For this review, take the finished solid that the model builds, in its own axes (mm). A direction names the side the tool comes from. Round coordinates to 2 decimals unless told otherwise and drop trailing zeros. Answer in a Markdown table with one row per item.
```python
from build123d import *

# Parameters (mm, degrees)
BOSS_EXTRUDE1_DEPTH     = 76.2
CUT_EXTRUDE1_DEPTH      = 79.288057838
CUT_EXTRUDE1_DEPTH_BACK = 79.288057838
SKETCH5_R               = 0.55245
SKETCH6_R               = 2.6035
CUT_EXTRUDE3_DEPTH      = 42.418


with BuildPart() as part:
    # Sketch4 → Boss-Extrude1 (new, symmetric)
    with BuildSketch(Plane.XY):
        with BuildLine():
            Line((4.190365, -12.7), (10.11729625, -12.7))
            ThreePointArc((10.11729625, -12.7), (11.943543585, -11.943543585), (12.7, -10.11729625))
            Line((12.7, -10.11729625), (12.7, -4.190365))
            ThreePointArc((12.7, -4.190365), (12.42492494, -3.52627506), (11.760835, -3.2512))
            Line((11.760835, -3.2512), (11.429365, -3.2512))
            ThreePointArc((11.429365, -3.2512), (10.76527506, -3.52627506), (10.4902, -4.190365))
            Line((10.4902, -4.190365), (10.4902, -6.348478019))
            ThreePointArc((10.4902, -6.348478019), (9.830707141, -7.335478831), (8.666460301, -7.103895736))
            Line((8.666460301, -7.103895736), (5.299899128, -3.737334563))
            ThreePointArc((5.299899128, -3.737334563), (4.817571085, -3.015479634), (4.6482, -2.16399369))
            Line((4.6482, -2.16399369), (4.6482, 0))
            Line((4.6482, 0), (2.6035, 0))
            ThreePointArc((2.6035, 0), (1.840952505, -1.840952505), (0, -2.6035))
            Line((0, -2.6035), (0, -4.6482))
            Line((0, -4.6482), (2.16399369, -4.6482))
            ThreePointArc((2.16399369, -4.6482), (3.015479634, -4.817571085), (3.737334563, -5.299899128))
            Line((3.737334563, -5.299899128), (7.103895736, -8.666460301))
            ThreePointArc((7.103895736, -8.666460301), (7.335478831, -9.830707141), (6.348478019, -10.4902))
            Line((6.348478019, -10.4902), (4.190365, -10.4902))
            ThreePointArc((4.190365, -10.4902), (3.52627506, -10.76527506), (3.2512, -11.429365))
            Line((3.2512, -11.429365), (3.2512, -11.760835))
            ThreePointArc((3.2512, -11.760835), (3.52627506, -12.42492494), (4.190365, -12.7))
        make_face()
    extrude(amount=BOSS_EXTRUDE1_DEPTH, both=True)

    # Sketch5 → Cut-Extrude1 (cut, two sides: drawn at the far end of the back side and taken through both)
    with BuildSketch(Plane.XY.offset(-CUT_EXTRUDE1_DEPTH_BACK)):
        with Locations((10.356153152, -12.7)):
            Circle(SKETCH5_R)
        with Locations((5.796028019, -12.7)):
            Circle(SKETCH5_R)
        with Locations((12.7, -10.356153152)):
            Circle(SKETCH5_R)
        with Locations((12.7, -5.796028019)):
            Circle(SKETCH5_R)
    extrude(amount=CUT_EXTRUDE1_DEPTH + CUT_EXTRUDE1_DEPTH_BACK, mode=Mode.SUBTRACT)

    # Mirror1: part across plane


with BuildPart() as part_1:
    add(part.part)
    add(part.part.mirror(Plane(origin=(0, 0, 0), x_dir=(0, 0, 1), z_dir=(1, 0, 0))))

    # Mirror2: part across plane


with BuildPart() as part_2:
    add(part_1.part)
    add(part_1.part.mirror(Plane.ZX))

    # Sketch6 → Cut-Extrude3 (cut)
    with BuildSketch(Plane.XY.offset(76.2)):
        with BuildLine():
            Line((12.7, -5.243578019), (12.7, -4.190365))
            ThreePointArc((12.7, -4.190365), (12.42492494, -3.52627506), (11.760835, -3.2512))
            Line((11.760835, -3.2512), (11.429365, -3.2512))
            ThreePointArc((11.429365, -3.2512), (10.76527506, -3.52627506), (10.4902, -4.190365))
            Line((10.4902, -4.190365), (10.4902, -6.348478019))
            ThreePointArc((10.4902, -6.348478019), (9.830707141, -7.335478831), (8.666460301, -7.103895736))
            Line((8.666460301, -7.103895736), (5.299899128, -3.737334563))
            ThreePointArc((5.299899128, -3.737334563), (4.817571085, -3.015479634), (4.6482, -2.16399369))
            Line((4.6482, -2.16399369), (4.6482, 2.16399369))
            ThreePointArc((4.6482, 2.16399369), (4.817571085, 3.015479634), (5.299899128, 3.737334563))
            Line((5.299899128, 3.737334563), (8.666460301, 7.103895736))
            ThreePointArc((8.666460301, 7.103895736), (9.830707141, 7.335478831), (10.4902, 6.348478019))
            Line((10.4902, 6.348478019), (10.4902, 4.190365))
            ThreePointArc((10.4902, 4.190365), (10.76527506, 3.52627506), (11.429365, 3.2512))
            Line((11.429365, 3.2512), (11.760835, 3.2512))
            ThreePointArc((11.760835, 3.2512), (12.42492494, 3.52627506), (12.7, 4.190365))
            Line((12.7, 4.190365), (12.7, 5.243578019))
            ThreePointArc((12.7, 5.243578019), (12.14755, 5.796028019), (12.7, 6.348478019))
            Line((12.7, 6.348478019), (12.7, 9.803703152))
            ThreePointArc((12.7, 9.803703152), (12.150857656, 10.295790178), (12.579996867, 10.895412135))
            ThreePointArc((12.579996867, 10.895412135), (11.943543585, 11.943543585), (10.895412135, 12.579996867))
            ThreePointArc((10.895412135, 12.579996867), (10.295790178, 12.150857656), (9.803703152, 12.7))
            Line((9.803703152, 12.7), (6.348478019, 12.7))
            ThreePointArc((6.348478019, 12.7), (5.796028019, 12.14755), (5.243578019, 12.7))
            Line((5.243578019, 12.7), (4.190365, 12.7))
            ThreePointArc((4.190365, 12.7), (3.52627506, 12.42492494), (3.2512, 11.760835))
            Line((3.2512, 11.760835), (3.2512, 11.429365))
            ThreePointArc((3.2512, 11.429365), (3.52627506, 10.76527506), (4.190365, 10.4902))
            Line((4.190365, 10.4902), (6.348478019, 10.4902))
            ThreePointArc((6.348478019, 10.4902), (7.335478831, 9.830707141), (7.103895736, 8.666460301))
            Line((7.103895736, 8.666460301), (3.737334563, 5.299899128))
            ThreePointArc((3.737334563, 5.299899128), (3.015479634, 4.817571085), (2.16399369, 4.6482))
            Line((2.16399369, 4.6482), (-2.16399369, 4.6482))
            ThreePointArc((-2.16399369, 4.6482), (-3.015479634, 4.817571085), (-3.737334563, 5.299899128))
            Line((-3.737334563, 5.299899128), (-7.103895736, 8.666460301))
            ThreePointArc((-7.103895736, 8.666460301), (-7.335478831, 9.830707141), (-6.348478019, 10.4902))
            Line((-6.348478019, 10.4902), (-4.190365, 10.4902))
            ThreePointArc((-4.190365, 10.4902), (-3.52627506, 10.76527506), (-3.2512, 11.429365))
            Line((-3.2512, 11.429365), (-3.2512, 11.760835))
            ThreePointArc((-3.2512, 11.760835), (-3.52627506, 12.42492494), (-4.190365, 12.7))
            Line((-4.190365, 12.7), (-5.243578019, 12.7))
            ThreePointArc((-5.243578019, 12.7), (-5.796028019, 12.14755), (-6.348478019, 12.7))
            Line((-6.348478019, 12.7), (-9.803703152, 12.7))
            ThreePointArc((-9.803703152, 12.7), (-10.295790178, 12.150857656), (-10.895412135, 12.579996867))
            ThreePointArc((-10.895412135, 12.579996867), (-11.943543585, 11.943543585), (-12.579996867, 10.895412135))
            ThreePointArc((-12.579996867, 10.895412135), (-12.150857656, 10.295790178), (-12.7, 9.803703152))
            Line((-12.7, 9.803703152), (-12.7, 6.348478019))
            ThreePointArc((-12.7, 6.348478019), (-12.14755, 5.796028019), (-12.7, 5.243578019))
            Line((-12.7, 5.243578019), (-12.7, 4.190365))
            ThreePointArc((-12.7, 4.190365), (-12.42492494, 3.52627506), (-11.760835, 3.2512))
            Line((-11.760835, 3.2512), (-11.429365, 3.2512))
            ThreePointArc((-11.429365, 3.2512), (-10.76527506, 3.52627506), (-10.4902, 4.190365))
            Line((-10.4902, 4.190365), (-10.4902, 6.348478019))
            ThreePointArc((-10.4902, 6.348478019), (-9.830707141, 7.335478831), (-8.666460301, 7.103895736))
            Line((-8.666460301, 7.103895736), (-5.299899128, 3.737334563))
            ThreePointArc((-5.299899128, 3.737334563), (-4.817571085, 3.015479634), (-4.6482, 2.16399369))
            Line((-4.6482, 2.16399369), (-4.6482, -2.16399369))
            ThreePointArc((-4.6482, -2.16399369), (-4.817571085, -3.015479634), (-5.299899128, -3.737334563))
            Line((-5.299899128, -3.737334563), (-8.666460301, -7.103895736))
            ThreePointArc((-8.666460301, -7.103895736), (-9.830707141, -7.335478831), (-10.4902, -6.348478019))
            Line((-10.4902, -6.348478019), (-10.4902, -4.190365))
            ThreePointArc((-10.4902, -4.190365), (-10.76527506, -3.52627506), (-11.429365, -3.2512))
            Line((-11.429365, -3.2512), (-11.760835, -3.2512))
            ThreePointArc((-11.760835, -3.2512), (-12.42492494, -3.52627506), (-12.7, -4.190365))
            Line((-12.7, -4.190365), (-12.7, -5.243578019))
            ThreePointArc((-12.7, -5.243578019), (-12.14755, -5.796028019), (-12.7, -6.348478019))
            Line((-12.7, -6.348478019), (-12.7, -9.803703152))
            ThreePointArc((-12.7, -9.803703152), (-12.150857656, -10.295790178), (-12.579996867, -10.895412135))
            ThreePointArc((-12.579996867, -10.895412135), (-11.943543585, -11.943543585), (-10.895412135, -12.579996867))
            ThreePointArc((-10.895412135, -12.579996867), (-10.295790178, -12.150857656), (-9.803703152, -12.7))
            Line((-9.803703152, -12.7), (-6.348478019, -12.7))
            ThreePointArc((-6.348478019, -12.7), (-5.796028019, -12.14755), (-5.243578019, -12.7))
            Line((-5.243578019, -12.7), (-4.190365, -12.7))
            ThreePointArc((-4.190365, -12.7), (-3.52627506, -12.42492494), (-3.2512, -11.760835))
            Line((-3.2512, -11.760835), (-3.2512, -11.429365))
            ThreePointArc((-3.2512, -11.429365), (-3.52627506, -10.76527506), (-4.190365, -10.4902))
            Line((-4.190365, -10.4902), (-6.348478019, -10.4902))
            ThreePointArc((-6.348478019, -10.4902), (-7.335478831, -9.830707141), (-7.103895736, -8.666460301))
            Line((-7.103895736, -8.666460301), (-3.737334563, -5.299899128))
            ThreePointArc((-3.737334563, -5.299899128), (-3.015479634, -4.817571085), (-2.16399369, -4.6482))
            Line((-2.16399369, -4.6482), (2.16399369, -4.6482))
            ThreePointArc((2.16399369, -4.6482), (3.015479634, -4.817571085), (3.737334563, -5.299899128))
            Line((3.737334563, -5.299899128), (7.103895736, -8.666460301))
            ThreePointArc((7.103895736, -8.666460301), (7.335478831, -9.830707141), (6.348478019, -10.4902))
            Line((6.348478019, -10.4902), (4.190365, -10.4902))
            ThreePointArc((4.190365, -10.4902), (3.52627506, -10.76527506), (3.2512, -11.429365))
            Line((3.2512, -11.429365), (3.2512, -11.760835))
            ThreePointArc((3.2512, -11.760835), (3.52627506, -12.42492494), (4.190365, -12.7))
            Line((4.190365, -12.7), (5.243578019, -12.7))
            ThreePointArc((5.243578019, -12.7), (5.796028019, -12.14755), (6.348478019, -12.7))
            Line((6.348478019, -12.7), (9.803703152, -12.7))
            ThreePointArc((9.803703152, -12.7), (10.295790178, -12.150857656), (10.895412135, -12.579996867))
            ThreePointArc((10.895412135, -12.579996867), (11.943543585, -11.943543585), (12.579996867, -10.895412135))
            ThreePointArc((12.579996867, -10.895412135), (12.150857656, -10.295790178), (12.7, -9.803703152))
            Line((12.7, -9.803703152), (12.7, -6.348478019))
            ThreePointArc((12.7, -6.348478019), (12.14755, -5.796028019), (12.7, -5.243578019))
        make_face()
        with Locations(Location((0, 0, 0), (0, 0, 180))):
            Circle(SKETCH6_R, mode=Mode.SUBTRACT)
    extrude(amount=-CUT_EXTRUDE3_DEPTH, mode=Mode.SUBTRACT)


solid = part_2.part
```
Q1. The part is to be moulded in two halves that separate along X. For faces 4 (the face through (10.49, -5, -20)), 5 (the face through (7.007, 5.444, -20.439)), 6 (the face through (8, -12.7, -20)), 7 (the face through (4.648, 0, -20)), say which applies: +X half, -X half, draft (parallel to the pull), parting line (faces both ways), or undercut.
Answer key:
| item | result |
|---|---|
| face 4 | undercut |
| face 5 | undercut |
| face 6 | draft |
| face 7 | +X half |
Q2. Tool access review of faces 1 (the face through (-4.648, 0, -20)), 2 (the face through (0, -4.648, -20)), 3 (the face through (-10.49, -5, -20)): name each direction out of +Z, -Z, +X, -X, +Y, -Y from which nothing blocks a thin tool from reaching the whole face with its end or side.
Answer key:
| item | result |
|---|---|
| face 1 | +Z, -Z, -X |
| face 2 | +Z, -Z, -Y |
| face 3 | +Z, -Z |
Q3. Clearance check with flat-ended pins moving along their axes: pin 1 Ø6 at (y, z) = (-10, -15) entering from -X; pin 2 Ø1.5 at (x, z) = (0.5, 21.5) entering from +Y; pin 3 Ø2 at (x, z) = (0.5, -14.5) entering from -Y. State where each tip first meets the part, or that it passes through.
Answer key:
| item | result |
|---|---|
| pin 1 | stops at x = -12.7 |
| pin 2 | stops at y = 4.65 |
| pin 3 | stops at y = -4.65 |
Q4. To check wall thickness, follow probe 1 along X at (y, z) = (5.75, -1.5); probe 2 along Y at (x, z) = (-7.25, -3); probe 3 along Y at (x, z) = (-6, 28.5). State the ranges of each line that lie inside material, in increasing order.
Answer key:
| item | result |
|---|---|
| probe 1 | x = -12.15 to -10.49, -7.31 to -4.19, 4.19 to 7.31, 10.49 to 12.15 |
| probe 2 | y = -12.7 to -10, -8.85 to -5.69, 5.69 to 8.85, 10 to 12.7 |
| probe 3 | y = -12.19 to -10.49, -7.56 to -4.44, 4.44 to 7.56, 10.49 to 12.19 |
